```python
from build123d import *

# Parameters (mm, degrees)
SKETCH9_R           = 9.525
CUT_EXTRUDE9_DEPTH  = 5.842
CUT_EXTRUDE10_START = 15.24
SKETCH10_R          = 9.525
CUT_EXTRUDE10_DEPTH = 15.24


with BuildPart() as part:
    # Sketch2 → Revolve2 (revolve)
    with BuildSketch(Plane.XY, mode=Mode.PRIVATE) as revolve2_sk:
        Polygon((0.078657589, 36.627682817), (0.078657589, 26.467682817), (19.690604477, 26.467682817), (19.690604477, 29.007682817), (5.162905757, 29.007682817), (5.162905757, 34.087682817), (19.690604477, 34.087682817), (19.690604477, 36.627682817), align=None)
        Polygon((207.088657589, 36.627682817), (19.690604477, 36.627682817), (19.690604477, 34.087682817), (204.548657589, 34.087682817), (204.548657589, 26.162), (226.138657589, 26.162), (226.138657589, 28.71633139), (207.088657589, 28.71633139), align=None)
        Polygon((19.690604477, 29.007682817), (19.690604477, 26.467682817), (199.468657589, 26.467682817), (199.468657589, 19.05), (226.138657589, 19.05), (226.138657589, 21.59), (202.008657589, 21.59), (202.008657589, 29.007682817), (127, 29.007682817), align=None)
    revolve(revolve2_sk.sketch.rotate(Axis((0, 0, 0), (1, 0, 0)), 90), axis=Axis((0, 0, 0), (1, 0, 0)))

    # Sketch9 → Cut-Extrude9 (cut)
    with BuildSketch(Plane(origin=(0, 36.627682817, 0), x_dir=(1, 0, 0), z_dir=(0, 1, 0))):
        with Locations(Location((23.718923994, 0, 0), (0, 0, 270))):
            Circle(SKETCH9_R)
    extrude(amount=-CUT_EXTRUDE9_DEPTH, mode=Mode.SUBTRACT)

    # Sketch10 → Cut-Extrude10 (cut)
    with BuildSketch(Plane(origin=(0, -36.627682817, 0), x_dir=(1, 0, 0), z_dir=(0, 1, 0)).offset(CUT_EXTRUDE10_START)):
        with Locations(Location((23.718923994, 0, 0), (0, 0, 270))):
            Circle(SKETCH10_R)
    extrude(amount=-CUT_EXTRUDE10_DEPTH, mode=Mode.SUBTRACT)


solid = part.part
```
Can you work these out from the model? Positions are in its coordinate system, mm. A direction names the side the tool comes from. Coordinates: 2 decimals unless noted, no trailing zeros. Write each loop counter-clockwise with the first axis right and the second up, starting at its lowest first coordinate (ties: lowest second). Pieces come first, ordered by that corner, then holes. Notation, with made-up numbers: (7, 36.25) - (30, 36.25) arc R33 ccw to (30, 70.25) - close; hole circle Ø9 at (-8.5, -12.75). An arc over 180 degrees is marked (long way). Return JSON: item names as keys, results as strings.
Q1. I'm going to push flat-ended pins straight in: pin 1 Ø3 at (x, y) = (142.5, -29) entering from -Z; pin 2 Ø8 at (y, z) = (27.5, 27.5) entering from +X; pin 3 Ø2 at (x, z) = (183, 25.5) entering from +Y. Where does each tip first touch, or does it pass through?
Computed values:
{"pin 1": "stops at z = -24.19", "pin 2": "stops at x = 207.09", "pin 3": "stops at y = 27.23"}
Q2. If we section it at D-D (z = 0): Count the separate pieces of the cut face and the enclosed holes in it, then the cut area to 3 significant figures.
Computed values:
{"separate pieces": "5", "enclosed holes": "0", "area": "2,280 mm2"}
Q3. Please list where these lines run through material, in increasing order: L1, parallel to Y at x = 214, z = 0; L2, parallel to Y at x = 146, z = 0; L3, parallel to X at y = 35.85, z = 0. Write a range as from..to.
Computed values:
{"L1": "y = -28.72..-26.16, -21.59..-19.05, 19.05..21.59, 26.16..28.72", "L2": "y = -36.63..-34.09, -29.01..-26.47, 26.47..29.01, 34.09..36.63", "L3": "x = 0.08..14.19, 33.24..207.09"}
Q4. If we section it at C-C (x = 164): Please give me the cut outline in (y, z).
Computed values:
{"outline": "circle Ø73.26 at (0, 0); circle Ø58.02 at (0, 0); hole circle Ø68.18 at (0, 0); hole circle Ø52.94 at (0, 0)"}
Q5. Thinking about a two-plate mould opening in X: for faces 1 (the flat face through (202.009, -22, 0)), 2 (the flat face through (207.089, 19, 22)), 3 (the cylindrical face through (212.99, 18.597, -4.13)), which applies, +X half, -X half, draft (parallel to the pull), parting line (faces both ways), or undercut?
Computed values:
{"face 1": "undercut", "face 2": "+X half", "face 3": "draft"}
Q6. On a 3-axis mill with a long thin cutter (end or side, diameter ignored), from which of +Z, -Z, +X, -X, +Y, -Y can I reach the whole of each face in a straight line? I mean faces 4 (the cylindrical face through (33.163, 34.706, -1.24)), 5 (the cylindrical face through (26.58, -34.652, 9.085)), 6 (the flat face through (199.469, 17, 11)), 7 (the cylindrical face through (106.25, 30.24, 15.73)), 8 (the cylindrical face through (213.905, -14.592, -15.913)). Say none if no direction works.
Computed values:
{"face 4": "+Y", "face 5": "-Y", "face 6": "-X", "face 7": "none", "face 8": "+X"}
